Could you check a few things on this model? Use its own coordinates, in mm. A direction names the side the tool comes from. Round coordinates to 2 decimals unless told otherwise and drop trailing zeros. Loops run counter-clockwise (first coordinate to the right, second up) from the corner with the lowest first, then second, coordinate; pieces in that order, holes last. Notation, with made-up numbers: (11, 24) -> (32, 24) arc R15 ccw to (32, 47) -> close; hole circle Ø5 at (33.25, 43.25). An arc over 180 degrees is marked (long way). Write each question's results on one line, items separated by ' | '. Start each with the question number.
1) If I drill on probe 1 along Y at (x, z) = (13, 6.75); probe 2 along X at (y, z) = (3.75, 2.75); probe 3 along Z at (x, y) = (-31, 4.5), over which ranges is the centre line in solid material (lowest first)?
2) Imagine slicing it at C-C, the plane x = -19. List the corners of the cut face in (y, z) for me.
3) Imagine slicing it at A-A, the plane x = 8. List the corners of the cut face in (y, z) for me, plus the area to 3 significant figures.
4) Imagine slicing it at B-B, the plane z = 6.25. List the corners of the cut face in (x, y) for me, plus the area to 3 significant figures.
5) Imagine slicing it at D-D, the plane y = -0.75. List the corners of the cut face in (x, z) for me.
6) We'd pull the mould along Y, two halves only. Please class faces 1 (the cylindrical face through (-33.5, -1.56, 1.95)), 2 (the conical face through (-39.59, -4.88, 0.43)), 3 (the cylindrical face through (24.699, 3.122, 0.285)), 4 (the conical face through (-39.57, 4.885, 0.418)): pulls with the +Y half, pulls with the -Y half, needs draft (parallel to the pull), parting line crosses it, or undercut.
7) For P1, Ø1.5, axis at x = 15.5, y = 0.5, coming from the -Z side, with a flat end and sliding along its axis, tell me the tip position at first contact or that it passes through.
8) Which directions (+Z, -Z, +X, -X, +Y, -Y) give clear straight access to the entire face, cutting with the end or side of a thin tool? Please do faces 5 (the flat face through (25, 2, 5)), 6 (the flat face through (7.4, -0.02, 8.63)), 7 (the flat face through (-37.19, -2.7, 1.5)).
from build123d import *

# Parameters (mm, degrees)
F1_DEPTH  = 10
F2_W      = 3
F2_H      = 7.3
F3_DEPTH  = 25.001
F5_DEPTH  = 10.001
F6_R      = 1
F8_DEPTH  = 1.5
F10_DEPTH = 25
F11_R     = 5
F12_SIZE  = 0.3


with BuildPart() as f1:
    # F0 (on Top) → F1 (new body)
    with BuildSketch(Plane.XY):
        Polygon((-40, 5), (-40, 1.5), (0, 1.5), (0, 0), (0, -1.5), (-40, -1.5), (-40, -5), (25, -5), (25, 0), (25, 5), align=None)
    extrude(amount=F1_DEPTH)

    # F2 (on face) → F3 (cut, through all)
    with BuildSketch(Plane(origin=(0, 0, 0), x_dir=(0, -1, 0), z_dir=(-1, 0, 0))):
        with Locations((0, 3.65)):
            Rectangle(F2_W, F2_H)
    extrude(amount=-F3_DEPTH, mode=Mode.SUBTRACT)

    # F4 (on face) → F5 (cut, through all)
    with BuildSketch(Plane.XZ.offset(5)):
        Polygon((-40, 10), (-40, 3), (5, 10), align=None)
    extrude(amount=-F5_DEPTH, mode=Mode.SUBTRACT)

    # F6
    f6_edges = [f1.edges().sort_by_distance(p)[0] for p in [
        (25, -3.25, 0),
        (25, 3.25, 0),
        (-40, -3.25, 0),
        (-40, 3.25, 0),
        (-40, -3.25, 3),
        (-40, 3.25, 3),
        (25, 0, 10),
    ]]
    fillet(f6_edges, radius=F6_R)

    # F7 (on Front) → F8 (cut, symmetric)
    with BuildSketch(Plane.XZ):
        Polygon((0, 10), (0, 7.3), (15, 10), align=None)
    extrude(amount=F8_DEPTH, both=True, mode=Mode.SUBTRACT)

    # F9 (on face) → F10 (cut)
    with BuildSketch(Plane(origin=(-1.4006750241, 0, 9.0043394407), x_dir=(0.988116469, 0, 0.1537070063), z_dir=(-0.1537070063, 0, 0.988116469))):
        Polygon((-28.2070668472, 0), (-38.2070668472, 3.25), (-47.1767681407, 6.1651529204), (-46.7135751583, -6.0146152011), (-38.2070668472, -3.25), align=None)
    extrude(amount=-F10_DEPTH, mode=Mode.SUBTRACT)

    # F11
    f11_edges = [f1.edges().sort_by_distance(p)[0] for p in [
        (-33.525134, 1.5, 1.979649),
        (-33.525134, -1.5, 1.979649),
    ]]
    fillet(f11_edges, radius=F11_R)

    # F12
    f12_edges = [f1.edges().sort_by_distance(p)[0] for p in [
        (-7.5, 5, 0),
        (24.707107, 5, 0.292893),
        (-39.707107, 5, 0.292893),
        (25, 5, 5),
        (-40, 5, 1.571765),
        (24.707107, 5, 9.707107),
        (-39.759509, 5, 2.794026),
        (14.5, 5, 10),
        (-17.076854, 5, 6.565823),
        (-7.5, -5, 0),
        (-39.707107, -5, 0.292893),
        (24.707107, -5, 0.292893),
        (-40, -5, 1.571765),
        (25, -5, 5),
        (-39.759509, -5, 2.794026),
        (24.707107, -5, 9.707107),
        (-17.076854, -5, 6.565823),
        (14.5, -5, 10),
    ]]
    chamfer(f12_edges, length=F12_SIZE)


solid = f1.part
Checked values:
1) probe 1: -5 to -1.5, 1.5 to 5 | probe 2: -39.8 to 25 | probe 3: 0 to 4.4
2) outline: (-5, 0.3) -> (-4.7, 0) -> (-1.5, 0) -> (-1.5, 6.27) -> (-4.7, 6.27) -> (-5, 5.96) -> close; (1.5, 0) -> (4.7, 0) -> (5, 0.3) -> (5, 5.96) -> (4.7, 6.27) -> (1.5, 6.27) -> close
3) outline: (-5, 0.3) -> (-4.7, 0) -> (-1.5, 0) -> (-1.5, 7.3) -> (1.5, 7.3) -> (1.5, 0) -> (4.7, 0) -> (5, 0.3) -> (5, 9.7) -> (4.7, 10) -> (1.5, 10) -> (1.5, 8.74) -> (-1.5, 8.74) -> (-1.5, 10) -> (-4.7, 10) -> (-5, 9.7) -> close | area: 74.1 mm^2
4) outline: (-19.11, -4.7) -> (-17.16, -5) -> (24.7, -5) -> (25, -4.7) -> (25, -1.5) -> (-19.11, -1.5) -> close; (-19.11, 1.5) -> (25, 1.5) -> (25, 4.7) -> (24.7, 5) -> (-17.16, 5) -> (-19.11, 4.7) -> close | area: 308 mm^2
5) outline: (0, 7.3) -> (25, 7.3) -> (25, 9) arc R1 ccw to (24, 10) -> (15, 10) -> close
6) face 1: undercut | face 2: pulls with the -Y half | face 3: needs draft | face 4: pulls with the +Y half
7) P1: z = 7.3
8) face 5: +Z, -Z, +X, +Y, -Y | face 6: +Z, -X | face 7: -Z, -X
